```python
from build123d import *

# Parameters (mm, degrees)
SKETCH3_R           = 3.175
SKETCH3_R_2         = 3.429
BOSS_EXTRUDE1_DEPTH = 27.94
CUT_EXTRUDE1_DEPTH  = 25.4
CHAMFER1_SIZE       = 0.254
CHAMFER2_SIZE       = 0.254


with BuildPart() as part:
    # Sketch3 → Boss-Extrude1 (new body)
    with BuildSketch(Plane.XY):
        with BuildLine():
            Line((107.95, -41.275), (-107.95, -41.275))
            ThreePointArc((-107.95, -41.275), (-112.440128061, -39.415128061), (-114.3, -34.925))
            Line((-114.3, -34.925), (-114.3, 34.925))
            ThreePointArc((-114.3, 34.925), (-112.440128061, 39.415128061), (-107.95, 41.275))
            Line((-107.95, 41.275), (107.95, 41.275))
            ThreePointArc((107.95, 41.275), (112.440128061, 39.415128061), (114.3, 34.925))
            Line((114.3, 34.925), (114.3, -34.925))
            ThreePointArc((114.3, -34.925), (112.440128061, -39.415128061), (107.95, -41.275))
        make_face()
        with Locations((-107.95, 34.925)):
            Circle(SKETCH3_R, mode=Mode.SUBTRACT)
        with Locations((-107.95, -34.925)):
            Circle(SKETCH3_R, mode=Mode.SUBTRACT)
        with Locations((107.95, -34.925)):
            Circle(SKETCH3_R, mode=Mode.SUBTRACT)
        with Locations((107.95, 34.925)):
            Circle(SKETCH3_R, mode=Mode.SUBTRACT)
        with Locations((-85.598, 0)):
            Circle(SKETCH3_R_2, mode=Mode.SUBTRACT)
        with Locations((85.598, 0)):
            Circle(SKETCH3_R_2, mode=Mode.SUBTRACT)
        with Locations((-15.875, 5.732638889)):
            Circle(SKETCH3_R, mode=Mode.SUBTRACT)
        with Locations((15.875, 5.732638889)):
            Circle(SKETCH3_R, mode=Mode.SUBTRACT)
        with Locations((15.875, -5.732638889)):
            Circle(SKETCH3_R, mode=Mode.SUBTRACT)
        with Locations((-15.875, -5.732638889)):
            Circle(SKETCH3_R, mode=Mode.SUBTRACT)
    extrude(amount=BOSS_EXTRUDE1_DEPTH)

    # Sketch4 → Cut-Extrude1 (cut)
    with BuildSketch(Plane.XY.offset(27.94)):
        with BuildLine():
            Line((107.95, 38.735), (-107.95, 38.735))
            ThreePointArc((-107.95, 38.735), (-110.644076836, 37.619076836), (-111.76, 34.925))
            Line((-111.76, 34.925), (-111.76, -34.925))
            ThreePointArc((-111.76, -34.925), (-110.644076836, -37.619076836), (-107.95, -38.735))
            Line((-107.95, -38.735), (107.95, -38.735))
            ThreePointArc((107.95, -38.735), (110.644076836, -37.619076836), (111.76, -34.925))
            Line((111.76, -34.925), (111.76, 34.925))
            ThreePointArc((111.76, 34.925), (110.644076836, 37.619076836), (107.95, 38.735))
        make_face()
    extrude(amount=-CUT_EXTRUDE1_DEPTH, mode=Mode.SUBTRACT)

    # Chamfer1
    chamfer1_edges = [part.edges().sort_by_distance(p)[0] for p in [
        (0, 41.275, 0),
        (112.440128061, 39.415128061, 0),
        (-89.027, 0, 0),
        (82.169, 0, 0),
        (-111.125, 34.925, 0),
        (-111.125, -34.925, 0),
        (104.775, -34.925, 0),
        (104.775, 34.925, 0),
        (-19.05, 5.732638889, 0),
        (12.7, 5.732638889, 0),
        (12.7, -5.732638889, 0),
        (-19.05, -5.732638889, 0),
        (114.3, 0, 0),
        (112.440128061, -39.415128061, 0),
        (0, -41.275, 0),
        (-112.440128061, -39.415128061, 0),
        (-114.3, 0, 0),
        (-112.440128061, 39.415128061, 0),
    ]]
    chamfer(chamfer1_edges, length=CHAMFER1_SIZE)

    # Chamfer2
    chamfer2_edges = [part.edges().sort_by_distance(p)[0] for p in [
        (111.76, 0, 2.54),
        (110.644076836, -37.619076836, 2.54),
        (0, -38.735, 2.54),
        (-110.644076836, -37.619076836, 2.54),
        (-111.76, 0, 2.54),
        (-110.644076836, 37.619076836, 2.54),
        (0, 38.735, 2.54),
        (110.644076836, 37.619076836, 2.54),
        (-89.027, 0, 2.54),
        (82.169, 0, 2.54),
        (-111.125, 34.925, 2.54),
        (-111.125, -34.925, 2.54),
        (104.775, -34.925, 2.54),
        (104.775, 34.925, 2.54),
        (-19.05, 5.732638889, 2.54),
        (12.7, 5.732638889, 2.54),
        (12.7, -5.732638889, 2.54),
        (-19.05, -5.732638889, 2.54),
    ]]
    chamfer(chamfer2_edges, length=CHAMFER2_SIZE)


solid = part.part
```
The model under review builds one solid part; all positions refer to its coordinate system, in mm. A direction names the side the tool comes from. Round coordinates to 2 decimals unless told otherwise and drop trailing zeros. Loops run counter-clockwise (first coordinate to the right, second up) from the corner with the lowest first, then second, coordinate; pieces in that order, holes last. Notation, with made-up numbers: M -32,21 L 5,21 A19 ccw 5,50 Z; hole C 32.5,87 d3. An arc over 180 degrees is marked long. Answer as a JSON object with one key per item and string values.
(1) Take a section at C-C on z = 15. Give the boundary of the cut face in (x, y) (3 decimals).
Resolved:
{"outline": "M -114.3,-34.925 A6.35 ccw -107.95,-41.275 L 107.95,-41.275 A6.35 ccw 114.3,-34.925 L 114.3,34.925 A6.35 ccw 107.95,41.275 L -107.95,41.275 A6.35 ccw -114.3,34.925 Z; hole M -111.76,-34.925 A3.81 ccw -107.95,-38.735 L 107.95,-38.735 A3.81 ccw 111.76,-34.925 L 111.76,34.925 A3.81 ccw 107.95,38.735 L -107.95,38.735 A3.81 ccw -111.76,34.925 Z"}
(2) To check wall thickness, follow line 1 along Y through (x, z) = (107.95, 0.9) (3 decimals); line 2 along Y through (x, z) = (9.5, 18) (3 decimals); line 3 along X through (y, z) = (31.5, 11.5). State the ranges of each line that lie inside material, in increasing order.
Resolved:
{"line 1": "-41.275 to -38.1, -31.75 to 31.75, 38.1 to 41.275", "line 2": "-41.275 to -38.735, 38.735 to 41.275", "line 3": "-114.3 to -111.76, 111.76 to 114.3"}
(3) Take a section at A-A on y = 0. Give the boundary of the cut face in (x, z) (3 decimals), and give its area (3 significant figures).
Resolved:
{"outline": "M -114.3,0.254 L -114.046,0 L -89.281,0 L -89.027,0.254 L -89.027,2.286 L -89.281,2.54 L -111.506,2.54 L -111.76,2.794 L -111.76,27.94 L -114.3,27.94 Z; M -82.169,0.254 L -81.915,0 L 81.915,0 L 82.169,0.254 L 82.169,2.286 L 81.915,2.54 L -81.915,2.54 L -82.169,2.286 Z; M 89.027,0.254 L 89.281,0 L 114.046,0 L 114.3,0.254 L 114.3,27.94 L 111.76,27.94 L 111.76,2.794 L 111.506,2.54 L 89.281,2.54 L 89.027,2.286 Z", "area": "675 mm²"}
(4) Draft analysis for pull direction Y (two halves, no side actions). For faces 3 (the conical face through (-112.4, 39.28, 0.13)), 4 (the flat face through (-2, -38.735, 16)), 5 (the flat face through (2, 1, 0)), state which applies: released by +Y, released by -Y, zero draft, split by the parting line, or undercut.
Resolved:
{"face 3": "released by +Y", "face 4": "undercut", "face 5": "zero draft"}
(5) Clearance check with flat-ended pins moving along their axes: P1, Ø7.5, axis at x = 107.95, y = 34.925, coming from the -Z side; P2, Ø6, axis at x = -56, y = 15, coming from the +Z side. State where each tip first meets the part, or that it passes through.
Resolved:
{"P1": "z = 0", "P2": "z = 2.54"}
(6) Take a section at D-D on y = 14. Give the boundary of the cut face in (x, z).
Resolved:
{"outline": "M -114.3,0.25 L -114.05,0 L 114.05,0 L 114.3,0.25 L 114.3,27.94 L 111.76,27.94 L 111.76,2.79 L 111.51,2.54 L -111.51,2.54 L -111.76,2.79 L -111.76,27.94 L -114.3,27.94 Z"}
(7) Take a section at B-B on x = -31.5. Give the boundary of the cut face in (y, z) (3 decimals).
Resolved:
{"outline": "M -41.275,0.254 L -41.021,0 L 41.021,0 L 41.275,0.254 L 41.275,27.94 L 38.735,27.94 L 38.735,2.794 L 38.481,2.54 L -38.481,2.54 L -38.735,2.794 L -38.735,27.94 L -41.275,27.94 Z"}
(8) Tool access review of faces 1 (the conical face through (-110.581, -37.499, 2.665)), 2 (the cylindrical face through (-106.24, 37.6, 1.26)): name each direction out of +Z, -Z, +X, -X, +Y, -Y from which nothing blocks a thin tool from reaching the whole face with its end or side.
Resolved:
{"face 1": "+Z", "face 2": "+Z, -Z"}
